```python
from build123d import *

# Parameters (mm, degrees)
ESQUISSE1_R               = 2
T_LE_DE_BASE_PLI_E1_DEPTH = 1.5
CONG_1_R                  = 3


# Sheet-metal steps are written as plain solids
with BuildPart() as part:
    # Esquisse1 → Tôle de base pliée1 (new body)
    with BuildSketch(Plane.XY):
        with BuildLine():
            Line((-8.5, 37.5), (8.5, 37.5))
            Line((8.5, 37.5), (8.5, -7.5))
            Line((8.5, -7.5), (-43.5, -7.5))
            ThreePointArc((-43.5, -7.5), (-50.393654271, -1.715537244), (-45.894141003, 6.077848346))
            Line((-45.894141003, 6.077848346), (-8.5, 19.688202607))
            Line((-8.5, 19.688202607), (-8.5, 37.5))
        make_face()
        with Locations((-43.5, -0.5)):
            Circle(ESQUISSE1_R, mode=Mode.SUBTRACT)
        with BuildLine():
            Line((1.75, 0.5), (1.75, -0.5))
            ThreePointArc((1.75, -0.5), (0, -2.25), (-1.75, -0.5))
            Line((-1.75, -0.5), (-1.75, 0.5))
            ThreePointArc((-1.75, 0.5), (0, 2.25), (1.75, 0.5))
        make_face(mode=Mode.SUBTRACT)
        with BuildLine():
            Line((1.75, 30.5), (1.75, 29.5))
            ThreePointArc((1.75, 29.5), (0, 27.75), (-1.75, 29.5))
            Line((-1.75, 29.5), (-1.75, 30.5))
            ThreePointArc((-1.75, 30.5), (0, 32.25), (1.75, 30.5))
        make_face(mode=Mode.SUBTRACT)
    extrude(amount=-T_LE_DE_BASE_PLI_E1_DEPTH)

    # Congé1
    cong_1_edges = [part.edges().sort_by_distance(p)[0] for p in [
        (-8.5, 37.5, -0.75),
        (8.5, 37.5, -0.75),
        (8.5, -7.5, -0.75),
        (-8.5, 19.688202607, -0.75),
    ]]
    fillet(cong_1_edges, radius=CONG_1_R)


solid = part.part
```
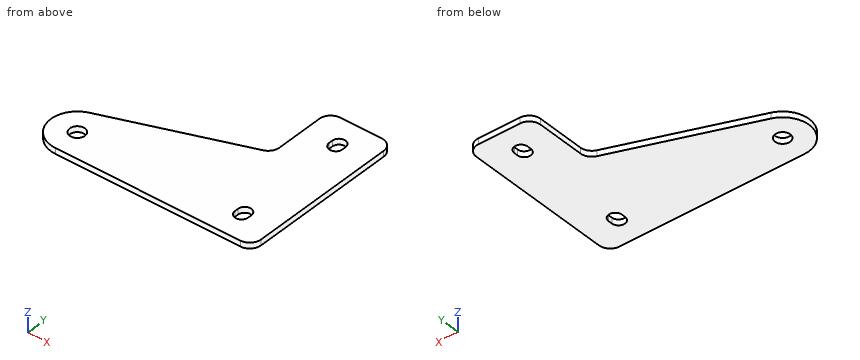
Design review of the part built by this model. Coordinates are the model's own, in mm. Round coordinates to 2 decimals unless told otherwise and drop trailing zeros. Write each loop counter-clockwise with the first axis right and the second up, starting at its lowest first coordinate (ties: lowest second). Pieces come first, ordered by that corner, then holes. Notation, with made-up numbers: (22, 21.25) -> (75, 21.25) arc R34 ccw to (75, 55.25) -> close; hole circle Ø2 at (71, -38). An arc over 180 degrees is marked (long way). Answer in a Markdown table with one row per item.
Q1. Take a section at A-A, the plane x = 0. State the section outline as (y, z) points.
The answers:
| item | result |
|---|---|
| outline | (-7.5, -1.5) -> (-2.25, -1.5) -> (-2.25, 0) -> (-7.5, 0) -> close; (2.25, -1.5) -> (27.75, -1.5) -> (27.75, 0) -> (2.25, 0) -> close; (32.25, -1.5) -> (37.5, -1.5) -> (37.5, 0) -> (32.25, 0) -> close |
Q2. Clearance check with a flat-ended pin moving along its axis: pin 1 Ø0.5 at (y, z) = (0, -1) entering from -X. State where the tip first meets the part, or that it passes through.
The answers:
| item | result |
|---|---|
| pin 1 | x = -50.5 |
Q3. Take a section at B-B, the plane z = -1.1. State the section outline as (x, y) points.
The answers:
| item | result |
|---|---|
| outline | (-45.89, 6.08) arc R7 ccw to (-43.5, -7.5) -> (5.5, -7.5) arc R3 ccw to (8.5, -4.5) -> (8.5, 34.5) arc R3 ccw to (5.5, 37.5) -> (-5.5, 37.5) arc R3 ccw to (-8.5, 34.5) -> (-8.5, 21.79) arc R3 cw to (-10.47, 18.97) -> close; hole circle Ø4 at (-43.5, -0.5); hole (-1.75, -0.5) arc R1.75 ccw to (1.75, -0.5) -> (1.75, 0.5) arc R1.75 ccw to (-1.75, 0.5) -> close; hole (-1.75, 29.5) arc R1.75 ccw to (1.75, 29.5) -> (1.75, 30.5) arc R1.75 ccw to (-1.75, 30.5) -> close |
Q4. To check wall thickness, follow L1, parallel to X at y = 30, z = -1.3; L2, parallel to Y at x = -0.5, z = -0.35; L3, parallel to X at y = 21.5, z = -0.9. State the ranges of each line that lie inside material, in increasing order. Write a range as [from, to].
The answers:
| item | result |
|---|---|
| L1 | [-8.5, -1.75], [1.75, 8.5] |
| L2 | [-7.5, -2.18], [2.18, 27.82], [32.18, 37.5] |
| L3 | [-8.51, 8.5] |
Q5. Take a section at C-C, the plane y = 26. State the section outline as (x, z) points.
The answers:
| item | result |
|---|---|
| outline | (-8.5, -1.5) -> (8.5, -1.5) -> (8.5, 0) -> (-8.5, 0) -> close |
Q6. Take a section at D-D, the plane x = -7.5. State the section outline as (y, z) points, then the cut area to 3 significant figures.
The answers:
| item | result |
|---|---|
| outline | (-7.5, -1.5) -> (36.74, -1.5) -> (36.74, 0) -> (-7.5, 0) -> close |
| area | 66.4 mm² |
